```python
from build123d import *

# Parameters (mm, degrees)
SKETCH_1_R          = 50
EXTRUDE_1_DEPTH     = 140
SKETCH_2_W          = 40
SKETCH_2_H          = 10
EXTRUDE_2_DEPTH     = 40
SKETCH_3_R          = 15
CUT_EXTRUDE_1_DEPTH = 40
EXTRUDE_4_DEPTH     = 10
FILLET_2_R          = 5


with BuildPart() as part:
    # 草圖1 → 填料-伸長1 (new body)
    with BuildSketch(Plane(origin=(0, 0, 0), x_dir=(1, 0, 0), z_dir=(0, 1, 0))):
        with Locations(Location((0, 0, 0), (0, 0, 270))):
            Circle(SKETCH_1_R)
    extrude(amount=EXTRUDE_1_DEPTH)

    # 草圖2 → 填料-伸長2 (add)
    with BuildSketch(Plane.XZ):
        with Locations((0, 50.82575695)):
            Rectangle(SKETCH_2_W, SKETCH_2_H)
    extrude(amount=-EXTRUDE_2_DEPTH)

    # 草圖3 → 除料-伸長1 (cut)
    with BuildSketch(Plane(origin=(0, 140, 0), x_dir=(1, 0, 0), z_dir=(0, 1, 0))):
        with Locations(Location((0, 0, 0), (0, 0, 270))):
            Circle(SKETCH_3_R)
    extrude(amount=-CUT_EXTRUDE_1_DEPTH, mode=Mode.SUBTRACT)

    # 草圖4 → 填料-伸長4 (add)
    with BuildSketch(Plane(origin=(0, 0, 0), x_dir=(0, 0, -1), z_dir=(1, 0, 0))):
        Polygon((-50, 140), (-60, 140), (-60, 130), (-50, 125), (-44.587553404, 125), (-44.587553404, 140), align=None)
    extrude(amount=EXTRUDE_4_DEPTH)

    # 圓角2
    fillet_2_edges = [part.edges().sort_by_distance(p)[0] for p in [
        (-5.0254481, 140, -49.74680765),
    ]]
    fillet(fillet_2_edges, radius=FILLET_2_R)


solid = part.part
```
Source: CAD feature listing. Evaluate the final solid. Frame: model axes, mm. A direction names the side the tool comes from. Give positions to 0.01 mm unless a question says otherwise; leave off trailing zeros. Loops run counter-clockwise (first coordinate to the right, second up) from the corner with the lowest first, then second, coordinate; pieces in that order, holes last. Notation, with made-up numbers: (85.5, 64.5) - (118.5, 64.5) arc R20 cw to (118.5, 69.5) - close; hole circle Ø1 at (-26, 1.25). An arc over 180 degrees is marked (long way). Use CSV: the item, a comma, the result in double quotes. Start each with the question number.
1. Section B-B (y = 120). Output: boundary loops of the cut face in (x, z).
2. Section A-A (z = 0). Output: boundary loops of the cut face in (x, y), then the cut area to 3 significant figures.
3. Draft query along Y for faces 1 (the flat face through (0, 40, 52)), 2 (the flat face through (-1, 140, -17)), 3 (the flat face through (20, 20, 51)), 4 (the flat face through (4.93, 127.535, 55.07)). Return one class per face: +Y half, -Y half, draft (parallel to the pull), parting line (faces both ways), or undercut.
4. Ray query, L1, parallel to Z at x = 1, y = 58; L2, parallel to Y at x = 5, z = 7; L3, parallel to X at y = 63.5, z = -26. Return the intervals inside material, ascending.
5. Section C-C (y = 81.5). Output: boundary loops of the cut face in (x, z).
6. Pin query (flat end, axial travel): pin 1 (1 mm diameter, centred on x = -28.5, z = 9, fed in from -Y); pin 2 (12 mm diameter, centred on y = 129.5, z = 49, fed in from +X); pin 3 (6 mm diameter, centred on y = 113.5, z = -15, fed in from -X); pin 4 (5 mm diameter, centred on x = -9.5, z = 49, fed in from +Y). Return the tip coordinate at first contact, or that it passes through.
7. Reachability of faces 5 (the flat face through (10, 134, 54)), 6 (the flat face through (-20, 20, 51)), 7 (the flat face through (0, 100, 0)) from +Z, -Z, +X, -X, +Y, -Y: full face, straight path, thin tool, end or side. Return the list, or none.
Response:
1,outline,"circle Ø100 at (0, 0); hole circle Ø30 at (0, 0)"
2,outline,"(-50, 0) - (50, 0) - (50, 135) arc R5 ccw to (45, 140) - (15, 140) - (15, 100) - (-15, 100) - (-15, 140) - (-45, 140) arc R5 ccw to (-50, 135) - close"
2,area,"12,800 mm²"
3,face 1,"undercut"
3,face 2,"+Y half"
3,face 3,"draft"
3,face 4,"undercut"
4,L1,"-49.99 to 49.99"
4,L2,"0 to 100"
4,L3,"-42.71 to 42.71"
5,outline,"circle Ø100 at (0, 0)"
6,pin 1,"y = 0"
6,pin 2,"x = 25.51"
6,pin 3,"x = -48.54"
6,pin 4,"y = 139.38"
7,face 5,"+Z, +X, +Y"
7,face 6,"+Z, -X, +Y, -Y"
7,face 7,"+Y"
